Can you work these out from the model? Positions are in its coordinate system, mm. A direction names the side the tool comes from. Round coordinates to 2 decimals unless told otherwise and drop trailing zeros. Use a Markdown table: item, result. Add a question column.
Q1. For faces 4 (the face through (-12.964, -6.015, 79.15)), 5 (the face through (73.304, 126, -2)), 6 (the face through (-68.862, 126, -3)), 7 (the face through (1, 126, 43.316)), which set-ups out of +Z, -Z, +X, -X, +Y, -Y let a thin tool reach every point of the face, with its end or its side?
Q2. We'd pull the mould along Y, two halves only. Please class faces 1 (the face through (3, 126, -47.759)), 2 (the face through (-1, 254, -1)), 3 (the face through (-22.025, 241.122, -99.184)): +Y half, -Y half, draft (parallel to the pull), parting line (faces both ways), or undercut.
Q3. I'm going to push flat-ended pins straight in: pin 1 Ø5.5 at (y, z) = (-7.5, 81) entering from -X; pin 2 Ø12 at (y, z) = (-3.5, 84) entering from +X. Where does each tip first touch, or does it pass through?
Q4. I need wall thicknesses on line 1 along Z through (x, y) = (54, 81); line 2 along Y through (x, z) = (-24, -41.5); line 3 along Z through (x, y) = (-201.5, -565). Which ranges of each line are inside material? Lowest first, please. Write a range as [from, to].
Autodesk Inventor part; units mm, degrees
ref_plane "Work Plane2" through (0, 0, 101.6) normal (0, -0.9659, 0.2588) x (1, 0, 0)
ref_plane "YZ Plane" through (0, 0, 0) normal (1, 0, 0) x (0, 1, 0)
ref_plane "XZ Plane" through (0, 0, 0) normal (0, 1, 0) x (-1, 0, 0)
sketch "Sketch1" plane through (0, 0, 0) normal (0, 1, 0) x (-1, 0, 0)
  circle A0 centre (0, 0) radius 101.6
  dimension "d0" = 203.2
extrude "Extrusion1" add sketch "Sketch1" along normal blind 25.4
sketch "Sketch2" plane through (0, 0, 0) normal (0, -1, 0) x (1, 0, 0)
  circle A0 centre (0, 0) radius 101.6
  point P0 (0, 101.6)
ref_plane "Work Plane1" through (0, 0, 101.6) normal (0, 0, 1) x (1, 0, 0)
sketch "Sketch3" plane through (0, 0, 101.6) normal (0, 0, 1) x (1, 0, 0)
  line L0 (0, 0) -> (50.8, 0) construction
  dimension "d3" = 50.8
ref_plane "Work Plane2" through (0, 0, 101.6) normal (0, -0.9659, 0.2588) x (1, 0, 0)
sketch "Sketch4" plane through (0, 0, 101.6) normal (0, -0.9659, 0.2588) x (1, 0, 0)
  line L0 (-19.0468, -4.4588) -> (19.0532, -4.4588)
  line L1 (19.0532, -4.4588) -> (19.0532, -42.5588)
  line L2 (19.0532, -42.5588) -> (-19.0468, -42.5588)
  line L3 (-19.0468, -42.5588) -> (-19.0468, -4.4588)
  point P0 (0, -98.1381)
  point P1 (0.0032, -0.0121)
  dimension "d5" = 38.1
  dimension "d6" = 38.1
extrude "Extrusion2" add sketch "Sketch4" against normal blind 25.4
sketch "Sketch5" plane through (0, 0, 101.6) normal (0, -0.9659, 0.2588) x (1, 0, 0)
  circle A0 centre (0, -23.5088) radius 12.7
  point P0 (0, -98.1381)
  dimension "d9" = 25.4
extrude "Extrusion3" add sketch "Sketch5" along normal blind 1270
pattern_circular "Circular Pattern2" count 3 over 360 about axis through (0, 0, 0) along (0, 1, 0) of "Extrusion2", "Extrusion3"
sketch "Sketch6" plane through (0, 25.4, 0) normal (0, 1, 0) x (1, 0, 0)
  line L0 (-68.8618, -43.3163) -> (73.3045, -43.3163)
  line L1 (73.3045, -43.3163) -> (73.3045, 47.759)
  line L2 (73.3045, 47.759) -> (-68.8618, 47.759)
  line L3 (-68.8618, 47.759) -> (-68.8618, -43.3163)
extrude "Extrusion4" add sketch "Sketch6" along normal blind 203.2
sketch "Sketch8" plane through (0, 228.6, 0) normal (0, 1, 0) x (1, 0, 0)
  circle A0 centre (0, 0) radius 101.6
  dimension "d23" = 203.2
extrude "Extrusion6" add sketch "Sketch8" along normal blind 25.4
properties part number "totalStation"
Answer below:
| question | item | result |
|---|---|---|
| 1 | face 4 | none |
| 1 | face 5 | +Z, -Z, +X |
| 1 | face 6 | +Z, -Z, -X |
| 1 | face 7 | +Z, +X, -X |
| 2 | face 1 | undercut |
| 2 | face 2 | +Y half |
| 2 | face 3 | draft |
| 3 | pin 1 | x = -19.05 |
| 3 | pin 2 | x = 63.73 |
| 4 | line 1 | [-47.76, 43.32] |
| 4 | line 2 | [0, 254] |
| 4 | line 3 | [-126.77, -102.09] |
